Geometry check sheet. Reference: the model listing, model coordinates, mm. Face numbers are marked on the shaded views. A direction names the side the tool comes from. Coordinates: 2 decimals unless noted, no trailing zeros. Loops run counter-clockwise (first coordinate to the right, second up) from the corner with the lowest first, then second, coordinate; pieces in that order, holes last.
Autodesk Inventor part; units mm, degrees
ref_plane "YZ Plane" through (0, 0, 0) normal (1, 0, 0) x (0, 1, 0)
ref_plane "XZ Plane" through (0, 0, 0) normal (0, 1, 0) x (-1, 0, 0)
ref_plane "XY Plane" through (0, 0, 0) normal (0, 0, 1) x (1, 0, 0)
sketch "Szkic1" plane through (0, 0, 0) normal (0, 0, 1) x (1, 0, 0)
  circle A0 centre (0, 0) radius 20
  circle A1 centre (0, 0) radius 20
  circle A2 centre (0, 0) radius 10
  point P0 (0, 0)
  dimension "d0" = 20
extrude "Wyciągnięcie proste1" add sketch "Szkic1" against normal blind 10
sketch "Szkic2" plane through (0, 0, 0) normal (0, 0, 1) x (1, 0, 0)
  circle A0 centre (0, 0) radius 20
  circle A1 centre (0, 0) radius 10
  circle A2 centre (0, 0) radius 25
  point P0 (0, 0)
  dimension "d3" = 50
extrude "Wyciągnięcie proste2" add sketch "Szkic2" along normal blind 30 contours A0 | A2
chamfer "Faza1" distance 1 angle 45 5 edges at (-25, 0, 0) (-20, 0, -10) (-10, 0, -10) (-25, 0, 30) (-10, 0, 30)
properties part number "uchwyt1" material "Rury z PCW"
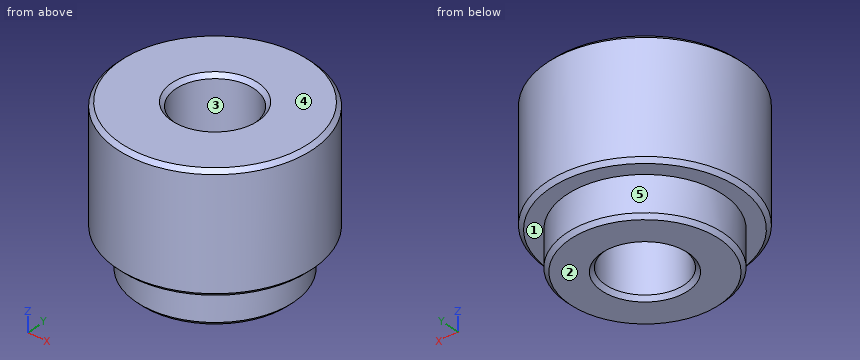
(1) Gauge pin test, flat ends, axial feed: pin 1 Ø3 at (x, z) = (-0.5, 25.5) entering from +Y; pin 2 Ø8 at (y, z) = (6, 11.5) entering from +X; pin 3 Ø4 at (x, z) = (18, -3.5) entering from -Y. Record the tip position at first contact, or that the pin passes through.
Findings:
pin 1: stops at y = 25
pin 2: stops at x = 24.92
pin 3: stops at y = -12
(2) Sectioned sample at A-A on x = 0. Record the cut outline in (y, z), and give its area (4 significant figures).
Findings:
outline: (-25, 1) - (-24, 0) - (-20, 0) - (-20, -9) - (-19, -10) - (-11, -10) - (-10, -9) - (-10, 29) - (-11, 30) - (-24, 30) - (-25, 29) - close; (10, -9) - (11, -10) - (19, -10) - (20, -9) - (20, 0) - (24, 0) - (25, 1) - (25, 29) - (24, 30) - (11, 30) - (10, 29) - close
area: 1,095 mm2
(3) Sectioned sample at D-D on z = -5. Record the cut outline in (x, y), and give its area (3 significant figures).
Findings:
outline: circle Ø40 at (0, 0); hole circle Ø20 at (0, 0)
area: 942 mm2
(4) Sectioned sample at C-C on z = 12. Record the cut outline in (x, y).
Findings:
outline: circle Ø50 at (0, 0); hole circle Ø20 at (0, 0)
(5) Scan lines: L1, parallel to Y at x = 0, z = 1; L2, parallel to X at y = -8, z = -5; L3, parallel to X at y = -8.5, z = -5. Record each from-to range of solid material in increasing order.
Findings:
L1: y = -25 to -10, 10 to 25
L2: x = -18.33 to -6, 6 to 18.33
L3: x = -18.1 to -5.27, 5.27 to 18.1
(6) Draft check along Y on the marked faces 3, 4 and 5. Enter one of: +Y half, -Y half, draft (parallel to the pull), parting line (faces both ways), or undercut.
Findings:
face 3: undercut
face 4: draft
face 5: parting line
(7) Access from +Z, -Z, +X, -X, +Y, -Y to the whole of each face (thin tool, end or side, straight path). Record for the marked faces 1 and 2.
Findings:
face 1: -Z
face 2: -Z, +X, -X, +Y, -Y
